```python
from build123d import *

# Parameters (mm, degrees)
MOUNT_DEPTH                      = 9.525
SKETCH2_W                        = 6.35
SKETCH2_H                        = 19.05
CENTER_CUTOUT_FOR_RIB_DEPTH      = 13.7
CENTER_CUTOUT_FOR_RIB_DEPTH_BACK = 13.7
SKETCH3_R                        = 3.175
PIN_HOLE_DEPTH                   = 10.525
PIN_HOLE_DEPTH_BACK              = 10.525


with BuildPart() as part:
    # Sketch1 → mount (new body, symmetric)
    with BuildSketch(Plane(origin=(0, 0, 0), x_dir=(0, 0, -1), z_dir=(1, 0, 0))):
        with BuildLine():
            Line((12.7, 0), (12.7, -12.7))
            ThreePointArc((12.7, -12.7), (0, -25.4), (-12.7, -12.7))
            Line((-12.7, -12.7), (-12.7, 0))
            Line((-12.7, 0), (12.7, 0))
        make_face()
    extrude(amount=MOUNT_DEPTH, both=True)

    # Sketch2 → center cutout for rib (cut, two sides)
    with BuildSketch(Plane.XY) as center_cutout_for_rib_sk:
        with Locations((0, -15.875)):
            Rectangle(SKETCH2_W, SKETCH2_H)
    extrude(amount=CENTER_CUTOUT_FOR_RIB_DEPTH, mode=Mode.SUBTRACT)
    extrude(center_cutout_for_rib_sk.sketch, amount=-CENTER_CUTOUT_FOR_RIB_DEPTH_BACK, mode=Mode.SUBTRACT)

    # Sketch3 → pin hole (cut, two sides)
    with BuildSketch(Plane(origin=(0, 0, 0), x_dir=(0, 0, -1), z_dir=(1, 0, 0))) as pin_hole_sk:
        with Locations((0, -12.7)):
            Circle(SKETCH3_R)
    extrude(amount=PIN_HOLE_DEPTH, mode=Mode.SUBTRACT)
    extrude(pin_hole_sk.sketch, amount=-PIN_HOLE_DEPTH_BACK, mode=Mode.SUBTRACT)


solid = part.part
```
Can you work these out from the model? Positions are in its coordinate system, mm. A direction names the side the tool comes from. Give positions to 0.01 mm unless a question says otherwise; leave off trailing zeros. Loops run counter-clockwise (first coordinate to the right, second up) from the corner with the lowest first, then second, coordinate; pieces in that order, holes last. Notation, with made-up numbers: M 83,-4.75 L 134,-4.75 A18 cw 134,10.25 Z; hole C 11.5,-2 d10. An arc over 180 degrees is marked long. Use one line per item in the form item = value. Start each with the question number.
(1) Please list where these lines run through material, in increasing order: line 1 (Z direction, x = 8.25, y = -12.7) (3 decimals); line 2 (Y direction, x = -5.5, z = 0) (3 decimals); line 3 (X direction, y = -22.5, z = -7.75) (3 decimals).
(2) On a 3-axis mill with a long thin cutter (end or side, diameter ignored), from which of +Z, -Z, +X, -X, +Y, -Y can I reach the whole of each face in a straight line? I mean faces 4 (the flat face through (0, -6, -12.7)), 5 (the flat face through (-3.175, -16, 3)). Say none if no direction works.
(3) Thinking about a two-plate mould opening in X: for faces 1 (the flat face through (9.525, -10, 3)), 2 (the flat face through (0, -6.35, 0)), 3 (the flat face through (0, 0, 0)), which applies, released by +X, released by -X, zero draft, split by the parting line, or undercut?
(4) I want a section at A-A, the plane z = 0. Write out the boundary of the cut face in (x, y) (3 decimals).
(5) I want a section at B-B, the plane y = -23.75. Write out the boundary of the cut face in (x, z) (3 decimals), and give its area (3 significant figures).
(6) I'm going to push flat-ended pins straight in: P1, Ø4, axis at x = 4, z = -4, coming from the +Y side; P2, Ø4, axis at y = -12.7, z = 0, coming from the +X side; P3, Ø3, axis at x = 1.5, z = 3.5, coming from the -Y side. Where does each tip first touch, or does it pass through?
(7) I want a section at C-C, the plane x = -7. Write out the boundary of the cut face in (y, z) (3 decimals), and give its area (3 significant figures).
(8) I want a section at D-D, the plane z = -5.5. Write out the boundary of the cut face in (x, y) (3 decimals), and give its area (3 significant figures).
Worked out:
q1.line_1 = -12.7 to -3.175, 3.175 to 12.7
q1.line_2 = -25.4 to -15.875, -9.525 to 0
q1.line_3 = -9.525 to -3.175, 3.175 to 9.525
q2.face_4 = -Z, +X, -X, +Y, -Y
q2.face_5 = +Z, -Z, -Y
q3.face_1 = released by +X
q3.face_2 = undercut
q3.face_3 = zero draft
q4.outline = M -9.525,-25.4 L -3.175,-25.4 L -3.175,-15.875 L -9.525,-15.875 Z; M -9.525,-9.525 L -3.175,-9.525 L -3.175,-6.35 L 3.175,-6.35 L 3.175,-9.525 L 9.525,-9.525 L 9.525,0 L -9.525,0 Z; M 3.175,-25.4 L 9.525,-25.4 L 9.525,-15.875 L 3.175,-15.875 Z
q5.outline = M -9.525,-6.26 L -3.175,-6.26 L -3.175,6.26 L -9.525,6.26 Z; M 3.175,-6.26 L 9.525,-6.26 L 9.525,6.26 L 3.175,6.26 Z
q5.area = 159 mm²
q6.P1 = 0
q6.P2 = through
q6.P3 = -6.35
q7.outline = M -12.7,-12.7 L 0,-12.7 L 0,12.7 L -12.7,12.7 A12.7 ccw Z; hole C -12.7,0 d6.35
q7.area = 544 mm²
q8.outline = M -9.525,-24.147 L -3.175,-24.147 L -3.175,-6.35 L 3.175,-6.35 L 3.175,-24.147 L 9.525,-24.147 L 9.525,0 L -9.525,0 Z
q8.area = 347 mm²
